from build123d import *

# Parameters (mm, degrees)
BASE_FLANGE1_DEPTH  = 3.175
FILLET1_R           = 25
SKETCH2_W           = 127
SKETCH2_H           = 50
CUT_EXTRUDE1_DEPTH  = 10
SKETCH3_W           = 100
SKETCH3_H           = 100
BOSS_EXTRUDE1_DEPTH = 2
SKETCH4_W           = 90
SKETCH4_H           = 90
BOSS_EXTRUDE2_DEPTH = 40
FILLET3_R           = 20


# Sheet-metal steps are written as plain solids
with BuildPart() as part:
    # Sketch1 → Base-Flange1 (new body)
    with BuildSketch(Plane.XY):
        Polygon((-305.02, 897.72), (-389.09, 263.21), (-290.03, 0), (290.03, 0), (389.09, 263.21), (305.02, 897.72), align=None)
    extrude(amount=-BASE_FLANGE1_DEPTH)

    # Fillet1
    fillet1_edges = [part.edges().sort_by_distance(p)[0] for p in [
        (-290.03, 0, -1.5875),
        (-389.09, 263.21, -1.5875),
        (-305.02, 897.72, -1.5875),
        (305.02, 897.72, -1.5875),
        (389.09, 263.21, -1.5875),
        (290.03, 0, -1.5875),
    ]]
    fillet(fillet1_edges, radius=FILLET1_R)

    # Sketch2 → Cut-Extrude1 (cut)
    with BuildSketch(Plane.XY):
        with Locations((-90, 535)):
            Rectangle(SKETCH2_W, SKETCH2_H)
        with Locations((90, 535)):
            Rectangle(SKETCH2_W, SKETCH2_H)
    extrude(amount=-CUT_EXTRUDE1_DEPTH, mode=Mode.SUBTRACT)

    # Sketch3 → Boss-Extrude1 (add)
    with BuildSketch(Plane(origin=(0, 0, -3.175), x_dir=(-1, 0, 0), z_dir=(0, 0, -1))):
        with Locations((0, 685)):
            Rectangle(SKETCH3_W, SKETCH3_H)
    extrude(amount=BOSS_EXTRUDE1_DEPTH)

    # Sketch4 → Boss-Extrude2 (add)
    with BuildSketch(Plane(origin=(0, 0, -5.175), x_dir=(-1, 0, 0), z_dir=(0, 0, -1))):
        with Locations((0, 685)):
            Rectangle(SKETCH4_W, SKETCH4_H)
    extrude(amount=BOSS_EXTRUDE2_DEPTH)

    # Fillet3
    fillet3_edges = [part.edges().sort_by_distance(p)[0] for p in [
        (-45, 685, -45.175),
        (0, 730, -45.175),
        (45, 685, -45.175),
        (0, 640, -45.175),
    ]]
    fillet(fillet3_edges, radius=FILLET3_R)


solid = part.part
Geometry: final body of the model. Coordinates: model frame, mm. A direction names the side the tool comes from. Round coordinates to 2 decimals unless told otherwise and drop trailing zeros. Order: outer loops, then holes, each group sorted by start corner. A loop starts at its lowest first (then second) coordinate and runs counter-clockwise, first axis right, second up.
Q1. Section C-C, the plane y = 67.5. Output: boundary loops of the cut face in (x, z) (3 decimals).
Result sheet:
outline: (-315.434, -3.175) - (315.434, -3.175) - (315.434, 0) - (-315.434, 0) - close
Q2. Pin query (flat end, axial travel): pin 1 (2 mm diameter, centred on x = -12.5, z = -4.5, fed in from -Y); pin 2 (3.5 mm diameter, centred on y = 528, z = -2.5, fed in from -X); pin 3 (2.5 mm diameter, centred on y = 533.5, z = -1, fed in from +X). Return the tip coordinate at first contact, or that it passes through.
Result sheet:
pin 1: stops at y = 635
pin 2: stops at x = -354.24
pin 3: stops at x = 353.44
Q3. Section A-A, the plane x = 9. Output: boundary loops of the cut face in (y, z) (3 decimals), and give its area (3 significant figures).
Result sheet:
outline: (0, -3.175) - (635, -3.175) - (635, -5.175) - (640, -5.175) - (640, -25.175) arc R20 ccw to (660, -45.175) - (710, -45.175) arc R20 ccw to (730, -25.175) - (730, -5.175) - (735, -5.175) - (735, -3.175) - (897.72, -3.175) - (897.72, 0) - (0, 0) - close
area: 6,480 mm2
Q4. Access query for faces 1 (the face through (-45, 684, -15)), 2 (the face through (1, 730, -15)), 3 (the face through (45, 684, -15)), 4 (the face through (1, 640, -15)). Directions: +Z, -Z, +X, -X, +Y, -Y. A direction counts if a zero-diameter tool reaches every point of the face in a straight line with its end or side. Return the directions, or none.
Result sheet:
face 1: -Z, -X, +Y, -Y
face 2: -Z, +X, -X, +Y
face 3: -Z, +X, +Y, -Y
face 4: -Z, +X, -X, -Y
Q5. Section B-B, the plane z = -13. Output: boundary loops of the cut face in (x, y).
Result sheet:
outline: (-45, 640) - (45, 640) - (45, 730) - (-45, 730) - close
Q6. Material intervals for probe 1 along Z at (x, y) = (118.5, 246) (3 decimals); probe 2 along Y at (x, z) = (-4, -25.5), sorted ascending.
Result sheet:
probe 1: z = -3.175 to 0
probe 2: y = 640 to 730
